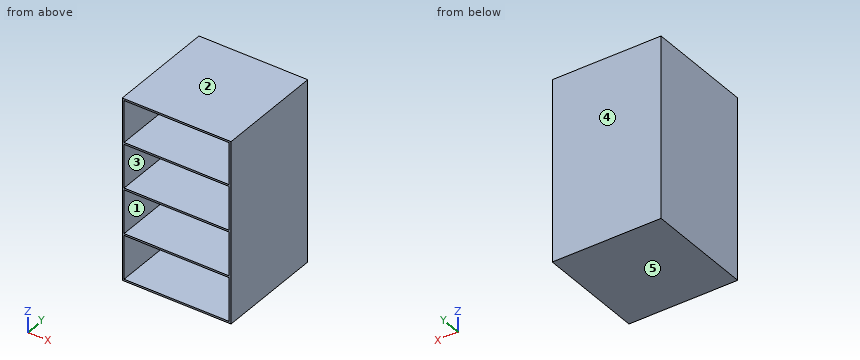
```python
from build123d import *

# Parameters (mm, degrees)
F0_W      = 60
F0_H      = 60
F1_DEPTH  = 50
F2_T      = -1
F5_W      = 60
F5_H      = 60
F6_DEPTH  = 1
F7_W      = 60
F7_H      = 60
F8_DEPTH  = 1
F9_W      = 60
F9_H      = 60
F10_DEPTH = 1


with BuildPart() as f1:
    # F0 (on Top) → F1 (new body, symmetric)
    with BuildSketch(Plane.XY):
        Rectangle(F0_W, F0_H)
    extrude(amount=F1_DEPTH, both=True)

    # F2
    f2_openings = [f1.faces().sort_by_distance(p)[0] for p in [
        (0, -30, 0),
    ]]
    offset(amount=F2_T, openings=f2_openings)

    # F5 (on offset) → F6 (join)
    with BuildSketch(Plane.XY.offset(25)):
        Rectangle(F5_W, F5_H)
    extrude(amount=F6_DEPTH)

    # F7 (on Top) → F8 (join)
    with BuildSketch(Plane.XY):
        Rectangle(F7_W, F7_H)
    extrude(amount=F8_DEPTH)

    # F9 (on offset) → F10 (join)
    with BuildSketch(Plane.XY.offset(-25)):
        Rectangle(F9_W, F9_H)
    extrude(amount=F10_DEPTH)


solid = f1.part
```
Geometry: final body of the model. Coordinates: model frame, mm. Face numbers are marked on the shaded views. A direction names the side the tool comes from. Round coordinates to 2 decimals unless told otherwise and drop trailing zeros. Loops run counter-clockwise (first coordinate to the right, second up) from the corner with the lowest first, then second, coordinate; pieces in that order, holes last. Notation, with made-up numbers: (10, 89) -> (58, 89) arc R21 ccw to (58, 123) -> close; hole circle Ø3 at (83, 10.5). An arc over 180 degrees is marked (long way). Use one line per item in the form item = value. Start each with the question number.
1) Section B-B on z = -11. Output: boundary loops of the cut face in (x, y), then the cut area to 3 significant figures.
2) Draft query along Z for the marked faces 3, 4 and 5. Return one class per face: released by +Z, released by -Z, zero draft, split by the parting line, or undercut.
3) Section A-A on y = 3. Output: boundary loops of the cut face in (x, z), then the cut area to 3 significant figures.
4) Line query: L1, parallel to Z at x = 25, y = -15; L2, parallel to X at y = -1, z = -10; L3, parallel to Y at x = 9, z = 19.5. Output: solid intervals per line, ascending.
5) Access query for the marked faces 1 and 2. Directions: +Z, -Z, +X, -X, +Y, -Y. A direction counts if a zero-diameter tool reaches every point of the face in a straight line with its end or side. Return the directions, or none.
6) Section C-C on x = 9.5. Output: boundary loops of the cut face in (y, z).
7) First-contact query: P1, Ø12, axis at x = -11.5, z = -9.5, coming from the -Y side. Flat tip, straight axial feed; report the tip coordinate or a pass-through.
Response:
q1.outline = (-30, -30) -> (-29, -30) -> (-29, 29) -> (29, 29) -> (29, -30) -> (30, -30) -> (30, 30) -> (-30, 30) -> close
q1.area = 178 mm^2
q2.face_3 = undercut
q2.face_4 = zero draft
q2.face_5 = released by -Z
q3.outline = (-30, -50) -> (30, -50) -> (30, 50) -> (-30, 50) -> close; hole (-29, -49) -> (29, -49) -> (29, -25) -> (-29, -25) -> close; hole (-29, -24) -> (29, -24) -> (29, 0) -> (-29, 0) -> close; hole (-29, 1) -> (29, 1) -> (29, 25) -> (-29, 25) -> close; hole (-29, 26) -> (29, 26) -> (29, 49) -> (-29, 49) -> close
q3.area = 490 mm^2
q4.L1 = -50 to -49, -25 to -24, 0 to 1, 25 to 26, 49 to 50
q4.L2 = -30 to -29, 29 to 30
q4.L3 = 29 to 30
q5.face_1 = -Y
q5.face_2 = +Z, +X, -X, +Y, -Y
q6.outline = (-30, -50) -> (30, -50) -> (30, 50) -> (-30, 50) -> (-30, 49) -> (29, 49) -> (29, 26) -> (-30, 26) -> (-30, 25) -> (29, 25) -> (29, 1) -> (-30, 1) -> (-30, 0) -> (29, 0) -> (29, -24) -> (-30, -24) -> (-30, -25) -> (29, -25) -> (29, -49) -> (-30, -49) -> close
q7.P1 = 29
